Study the drawing (mm; zero at the part's minimum x, y, z) and answer. Give positions to 0.01 mm unless a question says otherwise; leave off trailing zeros. Order: outer loops, then holes, each group sorted by start corner. A loop starts at its lowest first (then second) coordinate and runs counter-clockwise, first axis right, second up. Notation, with made-up numbers: (3.25, 70) - (35.25, 70) arc R23 ccw to (35.25, 101) - close; hole circle Ø4 at (30.5, -23). An arc over 180 degrees is marked (long way). Use CSV: the item, a comma, the result in double quotes.
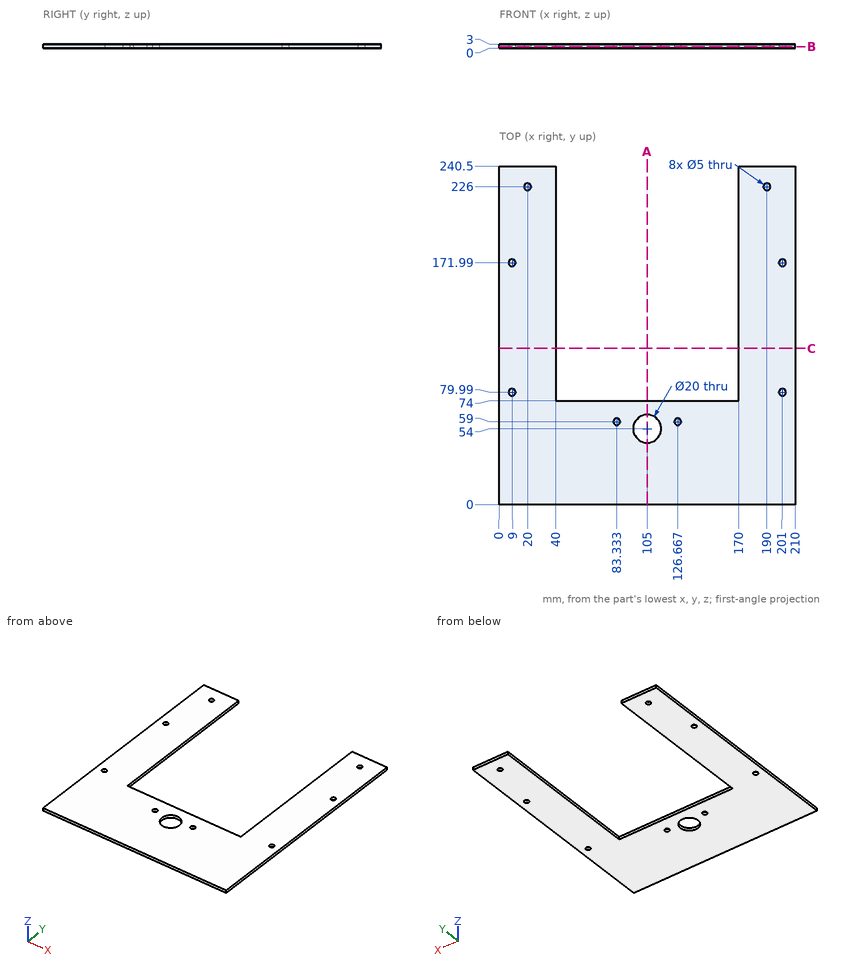
Item 1: The part is cut by section A-A (x = 105). Give the vertices of the cut face in (y, z).
Taken from the geometry:
outline,"(0, 0) - (44, 0) - (44, 3) - (0, 3) - close; (64, 0) - (74, 0) - (74, 3) - (64, 3) - close"
Item 2: The part is cut by section B-B (z = 1.05). Count the separate pieces of the cut face and the enclosed holes in it, and give its area (3 significant figures).
Taken from the geometry:
separate pieces,"1"
enclosed holes,"9"
area,"28,400 mm^2"
Item 3: This flat-tipped pin is pushed along its axis until it touches: pin 1 (3 mm diameter, centred on x = 190, y = 226, fed in from +Z). Where does it stop, or does it pass through?
Taken from the geometry:
pin 1,"through"
Item 4: The part is cut by section C-C (y = 111). Give the vertices of the cut face in (x, z), and give its area (3 significant figures).
Taken from the geometry:
outline,"(0, 0) - (40, 0) - (40, 3) - (0, 3) - close; (170, 0) - (210, 0) - (210, 3) - (170, 3) - close"
area,"240 mm^2"
Item 5: Find the intervals of material crossed by line 1 along Y through (x, z) = (9, 2.35); line 2 along X through (y, z) = (171.99, 2.4); line 3 along X through (y, z) = (121, 0.55), in increasing order.
Taken from the geometry:
line 1,"0 to 77.49, 82.49 to 169.49, 174.49 to 240.5"
line 2,"0 to 6.5, 11.5 to 40, 170 to 198.5, 203.5 to 210"
line 3,"0 to 40, 170 to 210"
